from build123d import *

# Parameters (mm, degrees)
SZKIC1_R                    = 8
DODANIE_WYCI_GNI_CIE1_DEPTH = 16
WYTNIJ_WYCI_GNI_CIE1_START  = -12
SZKIC2_R                    = 8
SZKIC2_R_2                  = 7
WYTNIJ_WYCI_GNI_CIE1_DEPTH  = 12
SZKIC3_R                    = 8
SZKIC3_R_2                  = 6.5
WYTNIJ_WYCI_GNI_CIE2_DEPTH  = 2


with BuildPart() as part:
    # Szkic1 → Dodanie-wyciągnięcie1 (new body)
    with BuildSketch(Plane.XY):
        Circle(SZKIC1_R)
    extrude(amount=DODANIE_WYCI_GNI_CIE1_DEPTH)

    # Szkic2 → Wytnij-wyciągnięcie1 (cut)
    with BuildSketch(Plane.XY.offset(16).offset(WYTNIJ_WYCI_GNI_CIE1_START)):
        Circle(SZKIC2_R)
        Circle(SZKIC2_R_2, mode=Mode.SUBTRACT)
    extrude(amount=WYTNIJ_WYCI_GNI_CIE1_DEPTH, mode=Mode.SUBTRACT)

    # Szkic3 → Wytnij-wyciągnięcie2 (cut)
    with BuildSketch(Plane(origin=(0, 0, 0), x_dir=(-1, 0, 0), z_dir=(0, 0, -1))):
        Circle(SZKIC3_R)
        Circle(SZKIC3_R_2, mode=Mode.SUBTRACT)
    extrude(amount=-WYTNIJ_WYCI_GNI_CIE2_DEPTH, mode=Mode.SUBTRACT)


solid = part.part
The listing builds one solid part. Answer for the finished solid, in the listing's coordinates (mm). A direction names the side the tool comes from. Round coordinates to 2 decimals unless told otherwise and drop trailing zeros. Write each loop counter-clockwise with the first axis right and the second up, starting at its lowest first coordinate (ties: lowest second). Pieces come first, ordered by that corner, then holes. Notation, with made-up numbers: (-17.5, 78.5) - (-11.5, 78.5) arc R7 ccw to (-11.5, 87.5) - close; hole circle Ø4 at (66, -7.75). An arc over 180 degrees is marked (long way). Use one line per item in the form item = value. Start each with the question number.
Item 1: A tool of negligible diameter and unlimited length cuts with its end or side. For faces 1 (the flat face through (0, 7, 2)), 2 (the cylindrical face through (-1.73, -7.81, 2.99)), 3 (the cylindrical face through (6.466, -2.681, 9.916)), from which of +Z, -Z, +X, -X, +Y, -Y can it reach the whole face along a straight path? Write none if from no direction.
Item 2: A cutting plane is placed at D-D (z = 2.5). Write down the section's boundary in (x, y), plus the area to 3 significant figures.
Item 3: A cutting plane is placed at A-A (x = 0). Write down the section's boundary in (y, z), plus the area to 3 significant figures.
Item 4: Find the intervals of material crossed by line 1 (Z direction, x = -5.25, y = 4); line 2 (Y direction, x = 0, z = 13); line 3 (Z direction, x = -6.75, y = 2.5), in increasing order. Write a range as [from, to].
Item 5: A cutting plane is placed at C-C (z = 5.25). Write down the section's boundary in (x, y), plus the area to 3 significant figures.
Item 6: Flat-ended cylindrical pins translate along their axes: pin 1 Ø8 at (x, z) = (-4, 11.5) entering from -Y; pin 2 Ø4 at (x, z) = (4.5, 3.5) entering from +Y; pin 3 Ø6 at (x, y) = (-0.5, 0) entering from -Z; pin 4 Ø1 at (y, z) = (2.5, 12) entering from +X. Find the tip coordinate at first contact, or state that the pin passes through.
The answers:
q1.face_1 = -Z
q1.face_2 = +Z, -Z
q1.face_3 = +Z
q2.outline = circle Ø16 at (0, 0)
q2.area = 201 mm^2
q3.outline = (-8, 2) - (-6.5, 2) - (-6.5, 0) - (6.5, 0) - (6.5, 2) - (8, 2) - (8, 4) - (7, 4) - (7, 16) - (-7, 16) - (-7, 4) - (-8, 4) - close
q3.area = 226 mm^2
q4.line_1 = [2, 16]
q4.line_2 = [-7, 7]
q4.line_3 = [2, 4]
q5.outline = circle Ø14 at (0, 0)
q5.area = 154 mm^2
q6.pin_1 = -7
q6.pin_2 = 7.6
q6.pin_3 = 0
q6.pin_4 = 6.71
